Verification items for the finished model (mm, model axes). Coordinates: 2 decimals unless noted, no trailing zeros.
Q1. Depth check by flat-ended pin: P1, Ø4, axis at x = -17.5, z = 7, coming from the -Y side; P2, Ø3, axis at x = -3, z = 9, coming from the +Y side; P3, Ø1, axis at y = -28, z = 3.5, coming from the +X side. Enter the tip coordinate at first touch or a pass-through.
Q2. Draft check along Y on faces 1 (the flat face through (-1, 11, 10)), 2 (the cylindrical face through (-8, 6, 5)). Enter one of: pulls with the +Y half, pulls with the -Y half, needs draft (parallel to the pull), parting line crosses it, or undercut.
Q3. Thickness scan on line 1 (Y direction, x = -38.5, z = 2); line 2 (X direction, y = -40.5, z = 8.75); line 3 (X direction, y = -5, z = 4). Record the ranges inside material, lowest first.
Q4. Cross-section at A-A, the plane y = -33. Count the separate pieces of the cut face and the enclosed holes in it, and give its area (3 significant figures).
from build123d import *

# Parameters (mm, degrees)
F1_DEPTH = 10


with BuildPart() as f1:
    # F0 (on Top) → F1 (new body)
    with BuildSketch(Plane.XY):
        with BuildLine():
            ThreePointArc((-10, 0), (0, 10), (10, 0))
            Line((10, 0), (36.3385102814, 0))
            add(Edge.make_bspline(
                [(36.3385102814, 0), (38.1493832545, 0.2133160809), (41.1543741544, 1.1173907107), (44.8944975107, 4.6532514581), (46.5891533047, 8.2707380904), (46.9314032298, 11.0166099485), (46.6155803767, 12.4906071166)],
                knots=[0, 0, 0, 0, 0.2631644028, 0.5247795892, 0.7588354663, 1, 1, 1, 1], degree=3))
            add(Edge.make_bspline(
                [(31.4700730394, 18.1692551407), (33.1449930775, 18.8899544822), (36.1994288499, 19.6094983358), (41.2064010634, 18.4174147824), (44.4827593479, 16.131907358), (46.1520924066, 13.9250375359), (46.6155803767, 12.4906071166)],
                knots=[0, 0, 0, 0, 0.2631644028, 0.5247795892, 0.7588354663, 1, 1, 1, 1], degree=3))
            add(Edge.make_bspline(
                [(31.4700730394, 18.1692551407), (32.9316769966, 19.2594287723), (35.0820381392, 21.5448758186), (36.5531496053, 26.4770827283), (36.2120212575, 30.4572459467), (35.135482458, 33.0063656939), (34.1249732601, 34.1249732601)],
                knots=[0, 0, 0, 0, 0.2631644028, 0.5247795892, 0.7588354663, 1, 1, 1, 1], degree=3))
            add(Edge.make_bspline(
                [(18.1692551407, 31.4700730394), (19.2594287723, 32.9316769966), (21.5448758186, 35.0820381392), (26.4770827283, 36.5531496053), (30.4572459467, 36.2120212575), (33.0063656939, 35.135482458), (34.1249732601, 34.1249732601)],
                knots=[0, 0, 0, 0, 0.2631644028, 0.5247795892, 0.7588354663, 1, 1, 1, 1], degree=3))
            add(Edge.make_bspline(
                [(18.1692551407, 31.4700730394), (18.8899544822, 33.1449930775), (19.6094983358, 36.1994288499), (18.4174147824, 41.2064010634), (16.131907358, 44.4827593479), (13.9250375359, 46.1520924066), (12.4906071166, 46.6155803767)],
                knots=[0, 0, 0, 0, 0.2631644028, 0.5247795892, 0.7588354663, 1, 1, 1, 1], degree=3))
            add(Edge.make_bspline(
                [(0, 36.3385102814), (0.2133160809, 38.1493832545), (1.1173907107, 41.1543741544), (4.6532514581, 44.8944975107), (8.2707380904, 46.5891533047), (11.0166099485, 46.9314032298), (12.4906071166, 46.6155803767)],
                knots=[0, 0, 0, 0, 0.2631644028, 0.5247795892, 0.7588354663, 1, 1, 1, 1], degree=3))
            add(Edge.make_bspline(
                [(0, 36.3385102814), (-0.2133160809, 38.1493832545), (-1.1173907107, 41.1543741544), (-4.6532514581, 44.8944975107), (-8.2707380904, 46.5891533047), (-11.0166099485, 46.9314032298), (-12.4906071166, 46.6155803767)],
                knots=[0, 0, 0, 0, 0.2631644028, 0.5247795892, 0.7588354663, 1, 1, 1, 1], degree=3))
            add(Edge.make_bspline(
                [(-18.1692551407, 31.4700730394), (-18.8899544822, 33.1449930775), (-19.6094983358, 36.1994288499), (-18.4174147824, 41.2064010634), (-16.131907358, 44.4827593479), (-13.9250375359, 46.1520924066), (-12.4906071166, 46.6155803767)],
                knots=[0, 0, 0, 0, 0.2631644028, 0.5247795892, 0.7588354663, 1, 1, 1, 1], degree=3))
            add(Edge.make_bspline(
                [(-18.1692551407, 31.4700730394), (-19.2594287723, 32.9316769966), (-21.5448758186, 35.0820381392), (-26.4770827283, 36.5531496053), (-30.4572459467, 36.2120212575), (-33.0063656939, 35.135482458), (-34.1249732601, 34.1249732601)],
                knots=[0, 0, 0, 0, 0.2631644028, 0.5247795892, 0.7588354663, 1, 1, 1, 1], degree=3))
            add(Edge.make_bspline(
                [(-31.4700730394, 18.1692551407), (-32.9316769966, 19.2594287723), (-35.0820381392, 21.5448758186), (-36.5531496053, 26.4770827283), (-36.2120212575, 30.4572459467), (-35.135482458, 33.0063656939), (-34.1249732601, 34.1249732601)],
                knots=[0, 0, 0, 0, 0.2631644028, 0.5247795892, 0.7588354663, 1, 1, 1, 1], degree=3))
            add(Edge.make_bspline(
                [(-31.4700730394, 18.1692551407), (-33.1449930775, 18.8899544822), (-36.1994288499, 19.6094983358), (-41.2064010634, 18.4174147824), (-44.4827593479, 16.131907358), (-46.1520924066, 13.9250375359), (-46.6155803767, 12.4906071166)],
                knots=[0, 0, 0, 0, 0.2631644028, 0.5247795892, 0.7588354663, 1, 1, 1, 1], degree=3))
            add(Edge.make_bspline(
                [(-36.3385102814, 0), (-38.1493832545, 0.2133160809), (-41.1543741544, 1.1173907107), (-44.8944975107, 4.6532514581), (-46.5891533047, 8.2707380904), (-46.9314032298, 11.0166099485), (-46.6155803767, 12.4906071166)],
                knots=[0, 0, 0, 0, 0.2631644028, 0.5247795892, 0.7588354663, 1, 1, 1, 1], degree=3))
            Line((-36.3385102814, 0), (-10, 0))
        make_face()
        with BuildLine():
            Line((36.3385102814, 0), (10, 0))
            ThreePointArc((10, 0), (0, -10), (-10, 0))
            Line((-10, 0), (-36.3385102814, 0))
            add(Edge.make_bspline(
                [(-36.3385102814, 0), (-38.1493832545, -0.2133160809), (-41.1543741544, -1.1173907107), (-44.8944975107, -4.6532514581), (-46.5891533047, -8.2707380904), (-46.9314032298, -11.0166099485), (-46.6155803767, -12.4906071166)],
                knots=[0, 0, 0, 0, 0.2631644028, 0.5247795892, 0.7588354663, 1, 1, 1, 1], degree=3))
            add(Edge.make_bspline(
                [(-31.4700730394, -18.1692551407), (-33.1449930775, -18.8899544822), (-36.1994288499, -19.6094983358), (-41.2064010634, -18.4174147824), (-44.4827593479, -16.131907358), (-46.1520924066, -13.9250375359), (-46.6155803767, -12.4906071166)],
                knots=[0, 0, 0, 0, 0.2631644028, 0.5247795892, 0.7588354663, 1, 1, 1, 1], degree=3))
            add(Edge.make_bspline(
                [(-31.4700730394, -18.1692551407), (-32.9316769966, -19.2594287723), (-35.0820381392, -21.5448758186), (-36.5531496053, -26.4770827283), (-36.2120212575, -30.4572459467), (-35.135482458, -33.0063656939), (-34.1249732601, -34.1249732601)],
                knots=[0, 0, 0, 0, 0.2631644028, 0.5247795892, 0.7588354663, 1, 1, 1, 1], degree=3))
            add(Edge.make_bspline(
                [(-18.1692551407, -31.4700730394), (-19.2594287723, -32.9316769966), (-21.5448758186, -35.0820381392), (-26.4770827283, -36.5531496053), (-30.4572459467, -36.2120212575), (-33.0063656939, -35.135482458), (-34.1249732601, -34.1249732601)],
                knots=[0, 0, 0, 0, 0.2631644028, 0.5247795892, 0.7588354663, 1, 1, 1, 1], degree=3))
            add(Edge.make_bspline(
                [(-18.1692551407, -31.4700730394), (-18.8899544822, -33.1449930775), (-19.6094983358, -36.1994288499), (-18.4174147824, -41.2064010634), (-16.131907358, -44.4827593479), (-13.9250375359, -46.1520924066), (-12.4906071166, -46.6155803767)],
                knots=[0, 0, 0, 0, 0.2631644028, 0.5247795892, 0.7588354663, 1, 1, 1, 1], degree=3))
            add(Edge.make_bspline(
                [(0, -36.3385102814), (-0.2133160809, -38.1493832545), (-1.1173907107, -41.1543741544), (-4.6532514581, -44.8944975107), (-8.2707380904, -46.5891533047), (-11.0166099485, -46.9314032298), (-12.4906071166, -46.6155803767)],
                knots=[0, 0, 0, 0, 0.2631644028, 0.5247795892, 0.7588354663, 1, 1, 1, 1], degree=3))
            add(Edge.make_bspline(
                [(0, -36.3385102814), (0.2133160809, -38.1493832545), (1.1173907107, -41.1543741544), (4.6532514581, -44.8944975107), (8.2707380904, -46.5891533047), (11.0166099485, -46.9314032298), (12.4906071166, -46.6155803767)],
                knots=[0, 0, 0, 0, 0.2631644028, 0.5247795892, 0.7588354663, 1, 1, 1, 1], degree=3))
            add(Edge.make_bspline(
                [(18.1692551407, -31.4700730394), (18.8899544822, -33.1449930775), (19.6094983358, -36.1994288499), (18.4174147824, -41.2064010634), (16.131907358, -44.4827593479), (13.9250375359, -46.1520924066), (12.4906071166, -46.6155803767)],
                knots=[0, 0, 0, 0, 0.2631644028, 0.5247795892, 0.7588354663, 1, 1, 1, 1], degree=3))
            add(Edge.make_bspline(
                [(18.1692551407, -31.4700730394), (19.2594287723, -32.9316769966), (21.5448758186, -35.0820381392), (26.4770827283, -36.5531496053), (30.4572459467, -36.2120212575), (33.0063656939, -35.135482458), (34.1249732601, -34.1249732601)],
                knots=[0, 0, 0, 0, 0.2631644028, 0.5247795892, 0.7588354663, 1, 1, 1, 1], degree=3))
            add(Edge.make_bspline(
                [(31.4700730394, -18.1692551407), (32.9316769966, -19.2594287723), (35.0820381392, -21.5448758186), (36.5531496053, -26.4770827283), (36.2120212575, -30.4572459467), (35.135482458, -33.0063656939), (34.1249732601, -34.1249732601)],
                knots=[0, 0, 0, 0, 0.2631644028, 0.5247795892, 0.7588354663, 1, 1, 1, 1], degree=3))
            add(Edge.make_bspline(
                [(31.4700730394, -18.1692551407), (33.1449930775, -18.8899544822), (36.1994288499, -19.6094983358), (41.2064010634, -18.4174147824), (44.4827593479, -16.131907358), (46.1520924066, -13.9250375359), (46.6155803767, -12.4906071166)],
                knots=[0, 0, 0, 0, 0.2631644028, 0.5247795892, 0.7588354663, 1, 1, 1, 1], degree=3))
            add(Edge.make_bspline(
                [(36.3385102814, 0), (38.1493832545, -0.2133160809), (41.1543741544, -1.1173907107), (44.8944975107, -4.6532514581), (46.5891533047, -8.2707380904), (46.9314032298, -11.0166099485), (46.6155803767, -12.4906071166)],
                knots=[0, 0, 0, 0, 0.2631644028, 0.5247795892, 0.7588354663, 1, 1, 1, 1], degree=3))
        make_face()
    extrude(amount=F1_DEPTH)


solid = f1.part
Check values:
1. P1: stops at y = -44.81
1. P2: stops at y = 44.43
1. P3: stops at x = 36.35
2. face 1: needs draft
2. face 2: undercut
3. line 1: y = -18.98 to -0.41, 0.41 to 18.98
3. line 2: x = -18.4 to -1.2, 1.2 to 18.4
3. line 3: x = -44.8 to -8.66, 8.66 to 44.8
4. separate pieces: 3
4. enclosed holes: 0
4. area: 685 mm2
